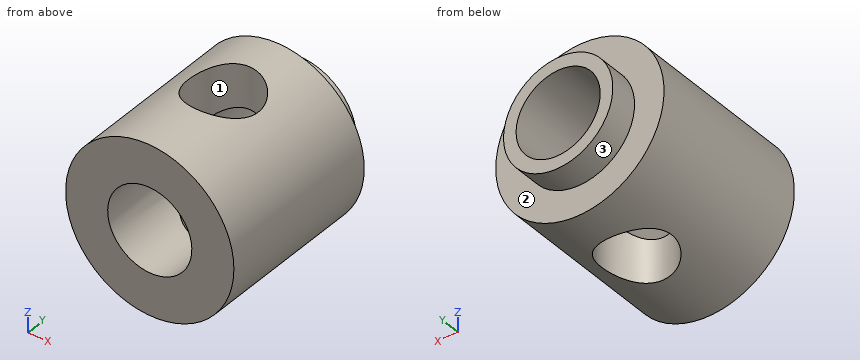
Autodesk Fusion 360 part; units mm, degrees
cylinder "CylinderPrimitive1" add diameter 6 height 6 placed x (1, 0, 0) y (0, 0, -1) z (0, 1, 0) at (0, 0, 0)
cylinder "CylinderPrimitive2" add diameter 3.9 height 1 placed x (1, 0, 0) y (0, 0, -1) z (0, 1, 0) at (0, 6, 0)
hole "Hole1" at (0, 7, 0) direction (0, -1, 0) diameter 3 end through all
hole "Hole2" at (0, 3.3861, 3) direction (0, 0, -1) diameter 2.5 depth 7 tip angle 118
Check sheet for the modelled part. Datum: model origin and axes. Units: mm. Face numbers are marked on the shaded views. Give positions to 0.01 mm unless a question says otherwise; leave off trailing zeros. Write each loop counter-clockwise with the first axis right and the second up, starting at its lowest first coordinate (ties: lowest second). Pieces come first, ordered by that corner, then holes. Notation, with made-up numbers: (-23, 31) - (-15, 31) arc R3 ccw to (-15, 35) - close; hole circle Ø2 at (28, 62.5). An arc over 180 degrees is marked (long way). Answer as a JSON object with one key per item and string values. Group by question number.
1) Thickness scan on probe 1 along Y at (x, z) = (0, 1.55); probe 2 along X at (y, z) = (4.25, 0); probe 3 along X at (y, z) = (5.25, -1.25). Record the ranges inside material, lowest first. Write a range as from..to.
2) Sectioned sample at D-D (y = 5.75). Record the cut outline in (x, z), then the cut area to 3 significant figures.
3) Release check for a two-part mould opening along Y. For the marked faces 1, 2 and 3 record: pulls with the +Y half, pulls with the -Y half, needs draft (parallel to the pull), parting line crosses it, or undercut.
4) Sectioned sample at B-B (x = 0). Record the cut outline in (y, z).
5) Sectioned sample at C-C (z = -1.75). Record the cut outline in (x, y).
6) Sectioned sample at A-A (z = 0). Record the cut outline in (x, y), then the cut area to 3 significant figures.
7) Depth check by flat-ended pin: P1, Ø1.5, axis at x = -1.5, y = 1.5, coming from the -Z side; P2, Ø1, axis at x = 2, y = 1.5, coming from the -Z side. Enter the tip coordinate at first touch or a pass-through.
Geometry results:
{
 "1": {"probe 1": "y = 0..2.14, 4.64..7", "probe 2": "x = -3..-1.5, 1.5..3", "probe 3": "x = -2.73..-0.83, 0.83..2.73"},
 "2": {"outline": "circle Ø6 at (0, 0); hole circle Ø3 at (0, 0)", "area": "21.2 mm^2"},
 "3": {"face 1": "undercut", "face 2": "pulls with the +Y half", "face 3": "needs draft"},
 "4": {"outline": "(0, -3) - (2.14, -3) - (2.14, -1.5) - (0, -1.5) - close; (0, 1.5) - (2.14, 1.5) - (2.14, 3) - (0, 3) - close; (4.64, -3) - (6, -3) - (6, -1.95) - (7, -1.95) - (7, -1.5) - (4.64, -1.5) - close; (4.64, 1.5) - (7, 1.5) - (7, 1.95) - (6, 1.95) - (6, 3) - (4.64, 3) - close"},
 "5": {"outline": "(-2.44, 0) - (2.44, 0) - (2.44, 6) - (0.86, 6) - (0.86, 7) - (-0.86, 7) - (-0.86, 6) - (-2.44, 6) - close; hole circle Ø2.5 at (0, 3.39)"},
 "6": {"outline": "(-3, 0) - (-1.5, 0) - (-1.5, 7) - (-1.95, 7) - (-1.95, 6) - (-3, 6) - close; (1.5, 0) - (3, 0) - (3, 6) - (1.95, 6) - (1.95, 7) - (1.5, 7) - close", "area": "18.9 mm^2"},
 "7": {"P1": "stops at z = -2.9", "P2": "stops at z = -2.6"}
}
